Input: part model. Units: mm. Frame: model coordinates. Coordinates: 2 decimals unless noted, no trailing zeros. Order: outer loops, then holes, each group sorted by start corner. A loop starts at its lowest first (then second) coordinate and runs counter-clockwise, first axis right, second up. Notation, with made-up numbers: (88, 89) -> (121, 89) arc R27 ccw to (121, 123) -> close; hole circle Ø1 at (-17.75, 60.25). An arc over 180 degrees is marked (long way). One line per question, with ' | ' between items.
```python
from build123d import *

# Parameters (mm, degrees)
F0_W     = 160
F0_H     = 8
F0_R     = 2.5
F1_DEPTH = 4
F2_R     = 2.5
F3_DEPTH = 8


with BuildPart() as f1:
    # F0 (on Top) → F1 (new body, symmetric)
    with BuildSketch(Plane.XY):
        Rectangle(F0_W, F0_H)
        with Locations((-76, 0)):
            Circle(F0_R, mode=Mode.SUBTRACT)
        with Locations((-68, 0)):
            Circle(F0_R, mode=Mode.SUBTRACT)
        with Locations((-60, 0)):
            Circle(F0_R, mode=Mode.SUBTRACT)
        with Locations((-52, 0)):
            Circle(F0_R, mode=Mode.SUBTRACT)
        with Locations((-44, 0)):
            Circle(F0_R, mode=Mode.SUBTRACT)
        with Locations((-36, 0)):
            Circle(F0_R, mode=Mode.SUBTRACT)
        with Locations((-28, 0)):
            Circle(F0_R, mode=Mode.SUBTRACT)
        with Locations((-20, 0)):
            Circle(F0_R, mode=Mode.SUBTRACT)
        with Locations((-12, 0)):
            Circle(F0_R, mode=Mode.SUBTRACT)
        with Locations((-4, 0)):
            Circle(F0_R, mode=Mode.SUBTRACT)
        with Locations((4, 0)):
            Circle(F0_R, mode=Mode.SUBTRACT)
        with Locations((12, 0)):
            Circle(F0_R, mode=Mode.SUBTRACT)
        with Locations((20, 0)):
            Circle(F0_R, mode=Mode.SUBTRACT)
        with Locations((28, 0)):
            Circle(F0_R, mode=Mode.SUBTRACT)
        with Locations((36, 0)):
            Circle(F0_R, mode=Mode.SUBTRACT)
        with Locations((44, 0)):
            Circle(F0_R, mode=Mode.SUBTRACT)
        with Locations((52, 0)):
            Circle(F0_R, mode=Mode.SUBTRACT)
        with Locations((60, 0)):
            Circle(F0_R, mode=Mode.SUBTRACT)
        with Locations((68, 0)):
            Circle(F0_R, mode=Mode.SUBTRACT)
        with Locations((76, 0)):
            Circle(F0_R, mode=Mode.SUBTRACT)
    extrude(amount=F1_DEPTH, both=True)

    # F2 (on face) → F3 (cut, through all)
    with BuildSketch(Plane.XZ.offset(4)):
        with Locations((-76, 0)):
            Circle(F2_R)
        with Locations((-68, 0)):
            Circle(F2_R)
        with Locations((-60, 0)):
            Circle(F2_R)
        with Locations((-52, 0)):
            Circle(F2_R)
        with Locations((-44, 0)):
            Circle(F2_R)
        with Locations((-36, 0)):
            Circle(F2_R)
        with Locations((-28, 0)):
            Circle(F2_R)
        with Locations((-20, 0)):
            Circle(F2_R)
        with Locations((-12, 0)):
            Circle(F2_R)
        with Locations((-4, 0)):
            Circle(F2_R)
        with Locations((4, 0)):
            Circle(F2_R)
        with Locations((12, 0)):
            Circle(F2_R)
        with Locations((20, 0)):
            Circle(F2_R)
        with Locations((28, 0)):
            Circle(F2_R)
        with Locations((36, 0)):
            Circle(F2_R)
        with Locations((44, 0)):
            Circle(F2_R)
        with Locations((52, 0)):
            Circle(F2_R)
        with Locations((60, 0)):
            Circle(F2_R)
        with Locations((68, 0)):
            Circle(F2_R)
        with Locations((76, 0)):
            Circle(F2_R)
    extrude(amount=-F3_DEPTH, mode=Mode.SUBTRACT)


solid = f1.part
```
1. Pin query (flat end, axial travel): pin 1 Ø4.5 at (x, z) = (28, 0) entering from +Y. Return the tip coordinate at first contact, or that it passes through.
Recorded:
pin 1: passes through
2. Mould query, pull axis Z, two halves, no side actions, for faces 1 (the face through (-78, 2.4, -1.5)), 2 (the face through (-22, -2.5, -1.5)), 3 (the face through (-1, 4, 0)). Classes: released by +Z, released by -Z, zero draft, split by the parting line, or undercut.
Recorded:
face 1: undercut | face 2: undercut | face 3: zero draft
3. Cut plane A-A, the plane x = -20. Return loops of the section in (y, z), and give its area (3 significant figures).
Recorded:
outline: (-4, -4) -> (-2.5, -4) -> (-2.5, -2.5) -> (-4, -2.5) -> close; (-4, 2.5) -> (-2.5, 2.5) -> (-2.5, 4) -> (-4, 4) -> close; (2.5, -4) -> (4, -4) -> (4, -2.5) -> (2.5, -2.5) -> close; (2.5, 2.5) -> (4, 2.5) -> (4, 4) -> (2.5, 4) -> close | area: 9.00 mm^2
4. Ray query, line 1 (Y direction, x = 58, z = -3.5); line 2 (Z direction, x = -44, y = 2.75). Return the intervals inside material, ascending. Write a range as [from, to].
Recorded:
line 1: y = [-4, -1.5], [1.5, 4] | line 2: z = [-4, -2.5], [2.5, 4]
